Here's the drawing with two shaded views (mm, measured from the low corner). I have some questions. A direction names the side the tool comes from. Round coordinates to 2 decimals unless told otherwise and drop trailing zeros. Order: outer loops, then holes, each group sorted by start corner. A loop starts at its lowest first (then second) coordinate and runs counter-clockwise, first axis right, second up.
Q1. If we section it at A-A (z = 38): Please give me the cut outline in (x, y).
Q2. If we section it at B-B (x = 5): Please give me the cut outline in (y, z), plus the area to 3 significant figures.
Q3. If I drill on line 1 (Z direction, x = 4.5, y = 0.75) (1 decimal); line 2 (Z direction, x = 6, y = 0.5); line 3 (Z direction, x = 16, y = 3.25), over which ranges is the centre line in solid material (lowest first)?
Q4. We'd pull the mould along X, two halves only. Please class the marked faces 1, 2 and 3: pulls with the +X half, pulls with the -X half, needs draft (parallel to the pull), parting line crosses it, or undercut.
Q5. For the marked faces 4 and 5, which set-ups out of +Z, -Z, +X, -X, +Y, -Y let a thin tool reach every point of the face, with its end or its side?
Q6. If we section it at C-C (y = 1.75): Please give me the cut outline in (x, z).
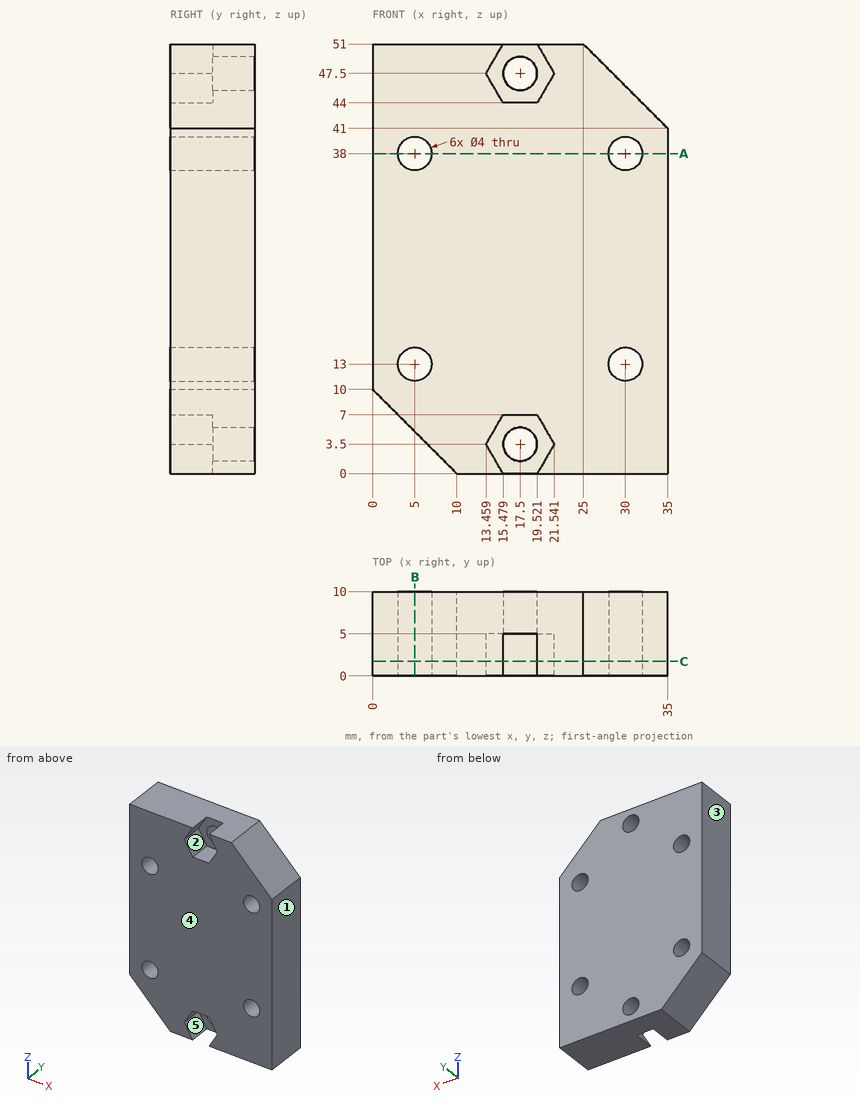
Solution:
1. outline: (0, 0) - (3, 0) - (3, 10) - (0, 10) - close; (7, 0) - (28, 0) - (28, 10) - (7, 10) - close; (32, 0) - (35, 0) - (35, 10) - (32, 10) - close
2. outline: (0, 5) - (10, 5) - (10, 11) - (0, 11) - close; (0, 15) - (10, 15) - (10, 36) - (0, 36) - close; (0, 40) - (10, 40) - (10, 51) - (0, 51) - close
2. area: 380 mm2
3. line 1: z = 5.5 to 11.1, 14.9 to 36.1, 39.9 to 51
3. line 2: z = 4 to 11.27, 14.73 to 36.27, 39.73 to 51
3. line 3: z = 7 to 44
4. face 1: pulls with the +X half
4. face 2: undercut
4. face 3: pulls with the -X half
5. face 4: +Z, -Z, +X, -X, -Y
5. face 5: -Y
6. outline: (0, 10) - (10, 0) - (15.48, 0) - (13.46, 3.5) - (15.48, 7) - (19.52, 7) - (21.54, 3.5) - (19.52, 0) - (35, 0) - (35, 41) - (25, 51) - (19.52, 51) - (21.54, 47.5) - (19.52, 44) - (15.48, 44) - (13.46, 47.5) - (15.48, 51) - (0, 51) - close; hole circle Ø4 at (5, 13); hole circle Ø4 at (5, 38); hole circle Ø4 at (30, 13); hole circle Ø4 at (30, 38)
